Model file for the job. Use its own axes, mm. Face numbers are marked on the shaded views. Round coordinates to 2 decimals unless told otherwise and drop trailing zeros. Write each loop counter-clockwise with the first axis right and the second up, starting at its lowest first coordinate (ties: lowest second). Pieces come first, ordered by that corner, then holes. Notation, with made-up numbers: (3.25, -17.75) - (33.25, -17.75) arc R14 ccw to (33.25, 6.25) - close; hole circle Ø7 at (27.25, 34.5). An arc over 180 degrees is marked (long way). One line per item, written item: value.
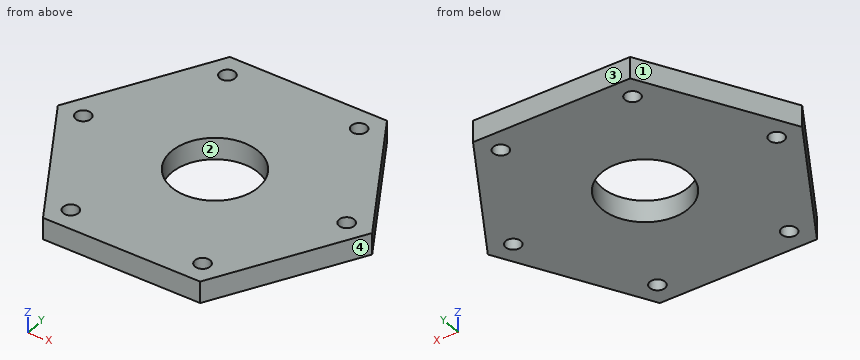
from build123d import *

# Parameters (mm, degrees)
F1_DEPTH = 5
F2_COUNT = 3
F3_R     = 10
F4_DEPTH = 5
F5_R     = 1.755872499
F6_DEPTH = 5


with BuildPart() as f1:
    # F0 (on Top) → F1 (new body)
    with BuildSketch(Plane.XY):
        Polygon((35.7957166898, 0), (17.8978583449, 31), (0, 0), (17.8978583449, -31), align=None)
    extrude(amount=-F1_DEPTH)

    # F2: F1 ×3 about axis
    f2_axis = Axis((0, 0, -2.5), (0, 0, 1))


with BuildPart() as f1_1:
    add(f1.part)
    for i in range(1, F2_COUNT):
        add(f1.part.rotate(f2_axis, i * 360 / F2_COUNT))

    # F3 (on face) → F4 (cut, through all)
    with BuildSketch(Plane.XY):
        Circle(F3_R)
    extrude(amount=-F4_DEPTH, mode=Mode.SUBTRACT)

    # F5 (on face) → F6 (cut, through all)
    with BuildSketch(Plane.XY):
        with Locations((15, -25.9807621135)):
            Circle(F5_R)
        with Locations((-15, -25.9807621135)):
            Circle(F5_R)
        with Locations((30, 0)):
            Circle(F5_R)
        with Locations((15, 25.9807621135)):
            Circle(F5_R)
        with Locations((-15, 25.9807621135)):
            Circle(F5_R)
        with Locations((-30, 0)):
            Circle(F5_R)
    extrude(amount=-F6_DEPTH, mode=Mode.SUBTRACT)


solid = f1_1.part
1. Band-saw the part on A-A on y = -6. Write the cut outline in (x, z).
Report:
outline: (-32.33, -5) - (-8, -5) - (-8, 0) - (-32.33, 0) - close; (8, -5) - (32.33, -5) - (32.33, 0) - (8, 0) - close
2. Wall check: probe 1 along Y at (x, z) = (15, -1.1); probe 2 along Y at (x, z) = (-13.5, -1.9); probe 3 along X at (y, z) = (-6, -3.9). Give the ranges that are in metal, low to high. Write a range as [from, to].
Report:
probe 1: [-31, -27.74], [-24.22, 24.22], [27.74, 31]
probe 2: [-31, -26.89], [-25.07, 25.07], [26.89, 31]
probe 3: [-32.33, -8], [8, 32.33]
3. Band-saw the part on B-B on x = 30. Write the cut outline in (y, z).
Report:
outline: (-10.04, -5) - (-1.76, -5) - (-1.76, 0) - (-10.04, 0) - close; (1.76, -5) - (10.04, -5) - (10.04, 0) - (1.76, 0) - close
4. Band-saw the part on C-C on z = -1.15. Write the cut outline in (x, y), plus the area to 3 significant figures.
Report:
outline: (-35.8, 0) - (-17.9, -31) - (17.9, -31) - (35.8, 0) - (17.9, 31) - (-17.9, 31) - close; hole circle Ø3.51 at (-30, 0); hole circle Ø3.51 at (-15, -25.98); hole circle Ø3.51 at (-15, 25.98); hole circle Ø20 at (0, 0); hole circle Ø3.51 at (15, -25.98); hole circle Ø3.51 at (15, 25.98); hole circle Ø3.51 at (30, 0)
area: 2,960 mm²
5. Band-saw the part on D-D on x = -15. Write the cut outline in (y, z).
Report:
outline: (-31, -5) - (-27.74, -5) - (-27.74, 0) - (-31, 0) - close; (-24.22, -5) - (24.22, -5) - (24.22, 0) - (-24.22, 0) - close; (27.74, -5) - (31, -5) - (31, 0) - (27.74, 0) - close
6. Drop flat-ended pins along their axis: pin 1 (1 mm diameter, centred on y = -10.5, z = -3, fed in from -X); pin 2 (3 mm diameter, centred on x = 30, y = 0, fed in from +Z); pin 3 (3 mm diameter, centred on x = 25.5, z = -1.5, fed in from +Y). Give the stop position or say it passes through.
Report:
pin 1: x = -30.02
pin 2: through
pin 3: y = 20.43
7. Mould opens along X. For the marked faces 1, 2, 3 and 4 say: released by +X, released by -X, zero draft, split by the parting line, or undercut.
Report:
face 1: released by -X
face 2: undercut
face 3: zero draft
face 4: released by +X
